```python
from build123d import *

# Parameters (mm, degrees)
SKETCH2_W                      = 30
SKETCH2_H                      = 45
BOSS_EXTRUDE1_DEPTH            = 9
SKETCH3_R                      = 11.05
CUT_EXTRUDE1_DEPTH             = 7
SKETCH4_R                      = 7.5
CUT_EXTRUDE2_DEPTH             = 28.932955447
FILLET1_R                      = 10
SKETCH5_W                      = 30
SKETCH5_H                      = 11
BOSS_EXTRUDE2_DEPTH            = 5.5
CBORE_FOR_M4_SHCS1_D           = 4.5
CBORE_FOR_M4_SHCS1_CBORE_D     = 8
CBORE_FOR_M4_SHCS1_CBORE_DEPTH = 4
RIB1_REACH                     = 37.387
SKETCH10_WALL_W                = 79.845356928
SKETCH10_WALL_H                = 4
F_3_3_3_3_DIAMETER_HOLE1_D     = 3.3
F_3_3_3_3_DIAMETER_HOLE1_DEPTH = 5
F_3_3_3_3_DIAMETER_HOLE1_TIP   = 0.991420021
SKETCH14_W                     = 30
SKETCH14_H                     = 5.5
BOSS_EXTRUDE3_DEPTH            = 11
MIRROR2_COPY_1_REACH           = 37.387
MIRROR2_COPY_1_SKETCH_W        = 79.845356928
MIRROR2_COPY_1_SKETCH_H        = 4


with BuildPart() as part:
    # Sketch2 → Boss-Extrude1 (new body)
    with BuildSketch(Plane(origin=(0, 0, 0), x_dir=(1, 0, 0), z_dir=(0, 1, 0))):
        Rectangle(SKETCH2_W, SKETCH2_H)
    extrude(amount=BOSS_EXTRUDE1_DEPTH)

    # Sketch3 → Cut-Extrude1 (cut)
    with BuildSketch(Plane(origin=(0, 9, 0), x_dir=(1, 0, 0), z_dir=(0, 1, 0))):
        with Locations(Location((0, 3.5, 0), (0, 0, 270))):
            Circle(SKETCH3_R)
    extrude(amount=-CUT_EXTRUDE1_DEPTH, mode=Mode.SUBTRACT)

    # Sketch4 → Cut-Extrude2 (cut, through all)
    with BuildSketch(Plane(origin=(0, 2, 0), x_dir=(1, 0, 0), z_dir=(0, 1, 0))):
        with Locations(Location((0, 3.5, 0), (0, 0, 270))):
            Circle(SKETCH4_R)
    extrude(amount=-CUT_EXTRUDE2_DEPTH, mode=Mode.SUBTRACT)

    # Fillet1
    fillet1_edges = [part.edges().sort_by_distance(p)[0] for p in [
        (-15, 4.5, -22.5),
        (15, 4.5, -22.5),
    ]]
    fillet(fillet1_edges, radius=FILLET1_R)

    # Sketch5 → Boss-Extrude2 (add)
    with BuildSketch(Plane.XY.offset(22.5)):
        with Locations((0, -5.5)):
            Rectangle(SKETCH5_W, SKETCH5_H)
    extrude(amount=-BOSS_EXTRUDE2_DEPTH)

    # CBORE for M4 SHCS1 (through all)
    with Locations(Plane(origin=(0, 0, 17), x_dir=(-1, 0, 0), z_dir=(0, 0, -1))):
        with Locations((0, -5.5)):
            cbore_for_m4_shcs1 = CounterBoreHole(CBORE_FOR_M4_SHCS1_D / 2, CBORE_FOR_M4_SHCS1_CBORE_D / 2, CBORE_FOR_M4_SHCS1_CBORE_DEPTH)

    # Sketch10 wall → Rib1 (add, up to next)
    with BuildSketch(Plane(origin=(-10, -2.5, 14.5), x_dir=(0, -0.707106781187, 0.707106781187), z_dir=(0, 0.707106781187, 0.707106781187)), mode=Mode.PRIVATE) as rib1_sk1:
        Rectangle(SKETCH10_WALL_W, SKETCH10_WALL_H)
    rib1_tool1 = extrude(rib1_sk1.sketch, amount=RIB1_REACH, mode=Mode.PRIVATE) - part.part
    rib1 = rib1_tool1.solids().sort_by_distance((-10, -2.5, 14.5))[0]
    add(rib1)

    # Mirror1: Rib1 across plane
    add(rib1.mirror(Plane(origin=(0, 0, 0), x_dir=(0, 0, 1), z_dir=(1, 0, 0))))

    # Ø3.3 (3.3) Diameter Hole1
    with Locations(Plane(origin=(0, 9, 0), x_dir=(1, 0, 0), z_dir=(0, 1, 0))):
        with Locations((0, -11.5), (0, 3.5), (0, 18.5)):
            Hole(F_3_3_3_3_DIAMETER_HOLE1_D / 2, depth=F_3_3_3_3_DIAMETER_HOLE1_DEPTH)
            with Locations((0, 0, -(F_3_3_3_3_DIAMETER_HOLE1_DEPTH + F_3_3_3_3_DIAMETER_HOLE1_TIP / 2))):  # 118° drill point
                Cone(0, F_3_3_3_3_DIAMETER_HOLE1_D / 2, F_3_3_3_3_DIAMETER_HOLE1_TIP, mode=Mode.SUBTRACT)

    # Sketch14 → Boss-Extrude3 (add)
    with BuildSketch(Plane(origin=(0, 9, 0), x_dir=(1, 0, 0), z_dir=(0, 1, 0))):
        with Locations((0, -19.75)):
            Rectangle(SKETCH14_W, SKETCH14_H)
    extrude(amount=BOSS_EXTRUDE3_DEPTH)

    # Mirror2: Rib1 across plane
    add(rib1.mirror(Plane(origin=(0, 4.5, 0), x_dir=(0, 0, 1), z_dir=(0, -1, 0))))

    # Mirror2 copy 1 sketch → Mirror2 copy 1 (add, up to next)
    with BuildSketch(Plane(origin=(10, 11.5, 14.5), x_dir=(0, 0.707106781187, 0.707106781187), z_dir=(0, -0.707106781187, 0.707106781187)), mode=Mode.PRIVATE) as mirror2_copy_1_sk1:
        Rectangle(MIRROR2_COPY_1_SKETCH_W, MIRROR2_COPY_1_SKETCH_H)
    mirror2_copy_1_tool1 = extrude(mirror2_copy_1_sk1.sketch, amount=MIRROR2_COPY_1_REACH, mode=Mode.PRIVATE) - part.part
    add(mirror2_copy_1_tool1.solids().sort_by_distance((10, 11.5, 14.5))[0])

    # Mirror3: CBORE for M4 SHCS1 across plane
    add(cbore_for_m4_shcs1.mirror(Plane(origin=(0, 4.5, 0), x_dir=(0, 0, 1), z_dir=(0, -1, 0))), mode=Mode.SUBTRACT)


solid = part.part
```
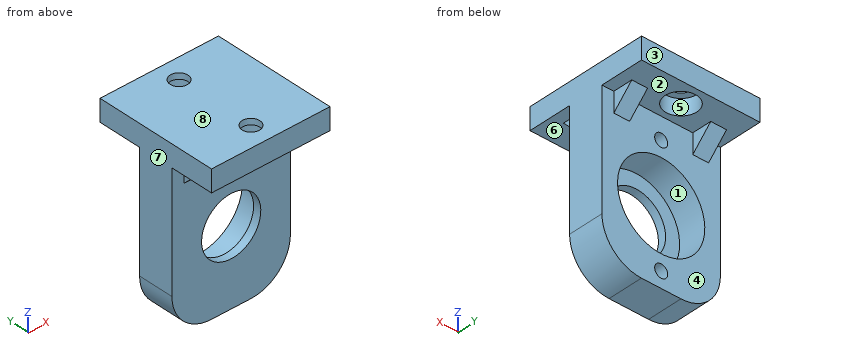
Model file for the job. Use its own axes, mm. Face numbers are marked on the shaded views. A direction names the side the tool comes from. Give positions to 0.01 mm unless a question says otherwise; leave off trailing zeros. Order: outer loops, then holes, each group sorted by start corner. A loop starts at its lowest first (then second) coordinate and runs counter-clockwise, first axis right, second up.
1) Saw through at D-D, the plane y = -5.5. Write the cut outline in (x, z), then the cut area to 3 significant figures.
2) Mould opens along Z. For the marked faces 1, 2 and 3 say: +Z half, -Z half, draft (parallel to the pull), parting line (faces both ways), or undercut.
3) 3-axis set-ups, long thin cutter, end or side, ignore diameter. For the marked faces 4, 5, 6, 7 and 8: which of +Z, -Z, +X, -X, +Y, -Y reach the whole face in a straight line?
4) Wall check: probe 1 along X at (y, z) = (14.5, 20.05); probe 2 along Y at (x, z) = (0, 19); probe 3 along Z at (x, y) = (-0.5, 7). Give the ranges that are in metal, low to high.
5) Saw through at A-A, the plane z = -3.5. Write the cut outline in (x, y), then the cut area to 3 significant figures.
6) Saw through at C-C, the plane x = 3. Write the cut outline in (y, z), then the cut area to 3 significant figures.
7) Pin check, flat tips, straight feed: pin 1 (1.5 mm diameter, centred on y = -2, z = 13.5, fed in from +X); pin 2 (9 mm diameter, centred on x = -6, y = 12.5, fed in from -Z); pin 3 (3.5 mm diameter, centred on x = -5.5, y = -3, fed in from -Z); pin 4 (4 mm diameter, centred on y = -2.5, z = 14.5, fed in from -X). Stop position of each tip, or through.
8) Saw through at B-B, the plane y = 4.5. Write the cut outline in (x, z).
Computed:
1. outline: (-15, 17) - (-4, 17) - (-4, 21) - (-2.25, 21) - (-2.25, 22.5) - (-15, 22.5) - close; (2.25, 21) - (4, 21) - (4, 17) - (15, 17) - (15, 22.5) - (2.25, 22.5) - close
1. area: 126 mm2
2. face 1: undercut
2. face 2: -Z half
2. face 3: draft
3. face 4: -Z, +Y
3. face 5: -Z
3. face 6: -Z, -Y
3. face 7: +Z, -Z, -X, +Y, -Y
3. face 8: +Z, +X, -X, +Y, -Y
4. probe 1: x = -15 to -4, 4 to 15
4. probe 2: y = -11 to -9.5, -1.5 to 10.5, 18.5 to 20
4. probe 3: z = -22.5 to -20.07, -16.93 to -14.54, 7.54 to 9.93, 13.07 to 22.5
5. outline: (-15, 0) - (-7.5, 0) - (-7.5, 2) - (-11.05, 2) - (-11.05, 9) - (-15, 9) - close; (7.5, 0) - (15, 0) - (15, 9) - (11.05, 9) - (11.05, 2) - (7.5, 2) - close
5. area: 85.3 mm2
6. outline: (-11, 17) - (-8.15, 17) - (-8.15, 21) - (-2.85, 21) - (-2.85, 17) - (0, 17) - (0, 3.37) - (2, 3.37) - (2, 7.13) - (9, 7.13) - (9, 17) - (11.85, 17) - (11.85, 21) - (17.15, 21) - (17.15, 17) - (20, 17) - (20, 22.5) - (-11, 22.5) - close; (0, -22.5) - (9, -22.5) - (9, -14.13) - (2, -14.13) - (2, -10.37) - (0, -10.37) - close
6. area: 307 mm2
7. pin 1: stops at x = 12
7. pin 2: stops at z = -22.5
7. pin 3: stops at z = 17
7. pin 4: stops at x = -12
8. outline: (-15, -12.5) arc R10 ccw to (-5, -22.5) - (5, -22.5) arc R10 ccw to (15, -12.5) - (15, 22.5) - (-15, 22.5) - close; hole circle Ø22.1 at (0, -3.5); hole circle Ø3.3 at (0, -18.5); hole circle Ø3.3 at (0, 11.5)
